For this review, use the dimensioned drawing (mm, ordinates from the lowest corner) and the shaded views. A direction names the side the tool comes from. Round coordinates to 2 decimals unless told otherwise and drop trailing zeros. Loops run counter-clockwise (first coordinate to the right, second up) from the corner with the lowest first, then second, coordinate; pieces in that order, holes last. Notation, with made-up numbers: M -23.75,56 L 8.25,56 A5 cw 8.25,65 Z; hole C 54,81.5 d9. An arc over 180 degrees is marked long. Write item = value, one per line. Start each with the question number.
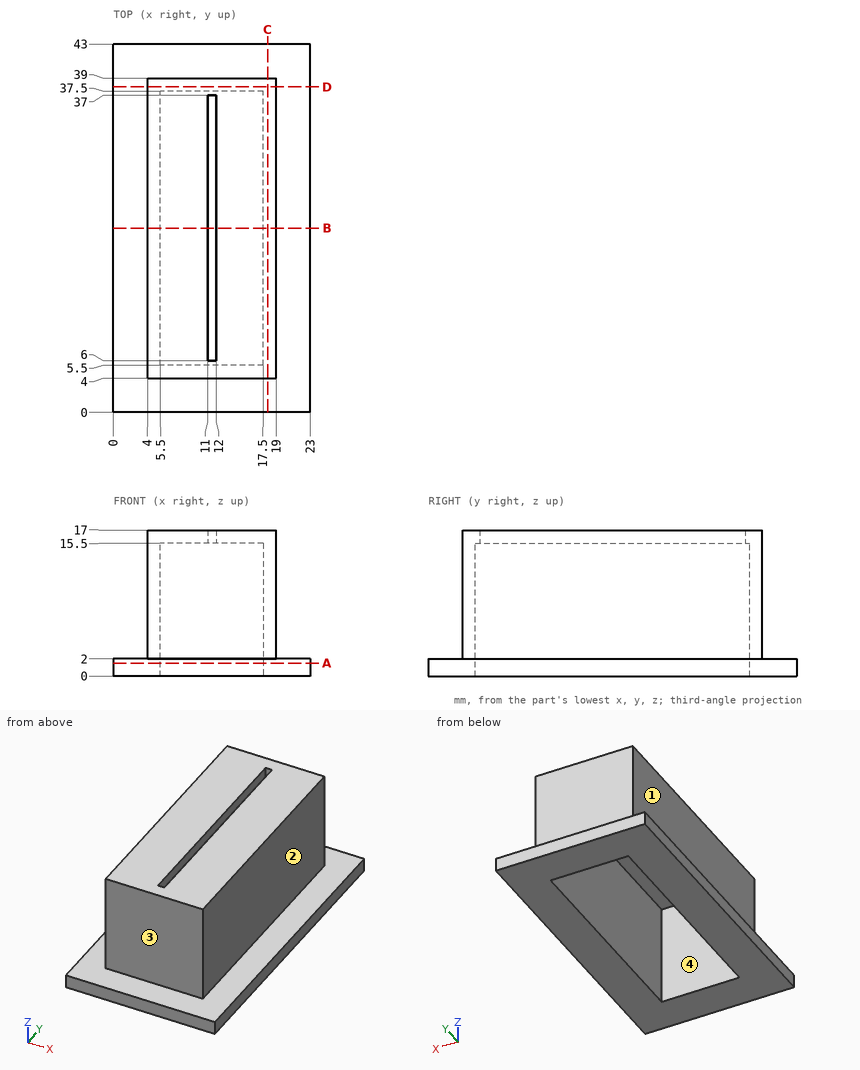
(1) Add section C-C on x = 18. Write out the cut boundary in (y, z), and give its area (3 significant figures).
(2) Add section D-D on y = 38. Write out the cut boundary in (x, z).
(3) For pin 1 Ø3.5 at (x, z) = (9, 5.5) entering from +Y; pin 2 Ø0.5 at (x, z) = (11.5, 16) entering from -Y; pin 3 Ø1.2 at (y, z) = (14, 16.5) entering from -X, all flat-tipped, find the tip position at first contact; note any pin that passes through.
(4) Wall thickness on L1, parallel to Y at x = 9.5, z = 4.5; L2, parallel to X at y = 34, z = 13; L3, parallel to X at y = 23.5, z = 1: over which ranges is each line inside the solid? List them lowest first.
(5) Tool access review of the marked faces 1, 2, 3 and 4: name each direction out of +Z, -Z, +X, -X, +Y, -Y from which nothing blocks a thin tool from reaching the whole face with its end or side.
(6) Add section A-A on z = 1.5. Write out the cut boundary in (x, y).
(7) Add section B-B on y = 21.5. Write out the cut boundary in (x, z), and give its area (3 significant figures).
Answer sheet:
q1.outline = M 0,0 L 43,0 L 43,2 L 39,2 L 39,17 L 4,17 L 4,2 L 0,2 Z
q1.area = 611 mm²
q2.outline = M 0,0 L 23,0 L 23,2 L 19,2 L 19,17 L 4,17 L 4,2 L 0,2 Z
q3.pin_1 = 39
q3.pin_2 = 4
q3.pin_3 = 4
q4.L1 = 4 to 5.5, 37.5 to 39
q4.L2 = 4 to 5.5, 17.5 to 19
q4.L3 = 0 to 5.5, 17.5 to 23
q5.face_1 = +Z, -X, +Y, -Y
q5.face_2 = +Z, +X, +Y, -Y
q5.face_3 = +Z, +X, -X, -Y
q5.face_4 = -Z
q6.outline = M 0,0 L 23,0 L 23,43 L 0,43 Z; hole M 5.5,5.5 L 17.5,5.5 L 17.5,37.5 L 5.5,37.5 Z
q7.outline = M 0,0 L 5.5,0 L 5.5,15.5 L 11,15.5 L 11,17 L 4,17 L 4,2 L 0,2 Z; M 12,15.5 L 17.5,15.5 L 17.5,0 L 23,0 L 23,2 L 19,2 L 19,17 L 12,17 Z
q7.area = 83.5 mm²
